from build123d import *

# Parameters (mm, degrees)
F0_R     = 10
F0_W     = 5
F0_H     = 8
F0_W_2   = 8
F0_H_2   = 5
F0_R_2   = 5
F1_DEPTH = 25


with BuildPart() as f1:
    # F0 (on Front) → F1 (new body)
    with BuildSketch(Plane.XZ):
        with BuildLine():
            ThreePointArc((60.975433, 96.400047), (60.980972, 96.732847), (60.982819, 97.065687))
            ThreePointArc((60.982819, 97.065687), (35.755982, 126.683535), (2.501691, 106.49041))
            ThreePointArc((2.501691, 106.49041), (2.393928, 106.15023), (2.285558, 105.810243))
            ThreePointArc((2.285558, 105.810243), (4.350114, 83.256305), (21.59361, 68.572833))
            ThreePointArc((21.59361, 68.572833), (48.295056, 72.564944), (60.975433, 96.400047))
        make_face()
        with Locations((30.982819, 97.065687)):
            Circle(F0_R, mode=Mode.SUBTRACT)
        with BuildLine():
            ThreePointArc((2.285558, 105.810243), (2.393928, 106.15023), (2.501691, 106.49041))
            ThreePointArc((2.501691, 106.49041), (2.391602, 106.150969), (2.285558, 105.810243))
        make_face()
        with BuildLine():
            ThreePointArc((-2.732649, -90.243404), (53.726427, -5.320256), (60.975433, 96.400047))
            ThreePointArc((60.975433, 96.400047), (48.295056, 72.564944), (21.59361, 68.572833))
            ThreePointArc((21.59361, 68.572833), (4.350114, 83.256305), (2.285558, 105.810243))
            ThreePointArc((2.285558, 105.810243), (-33.312028, 40.206629), (-90.483698, -7.776936))
            ThreePointArc((-90.483698, -7.776936), (-60.597191, -3.648374), (-33.776396, -17.46479))
            ThreePointArc((-33.776396, -17.46479), (-23.661975, -19.395325), (-14.685962, -14.349569))
            ThreePointArc((-14.685962, -14.349569), (-0.249152, -19.279648), (-7.475156, -32.715124))
            ThreePointArc((-7.475156, -32.715124), (-14.965806, -40.251179), (-25.569357, -40.934313))
            ThreePointArc((-25.569357, -40.934313), (-34.054638, -44.449031), (-37.569357, -52.934313))
            ThreePointArc((-37.569357, -52.934313), (-34.054638, -61.419594), (-25.569357, -64.934313))
            ThreePointArc((-25.569357, -64.934313), (-14.965806, -65.617446), (-7.475156, -73.153501))
            ThreePointArc((-7.475156, -73.153501), (0.078463, -80.260328), (-2.732649, -90.243404))
        make_face()
        with BuildLine():
            ThreePointArc((-3.124438, -90.590489), (-2.92843, -90.417074), (-2.732649, -90.243404))
            ThreePointArc((-2.732649, -90.243404), (0.078463, -80.260328), (-7.475156, -73.153501))
            ThreePointArc((-7.475156, -73.153501), (-14.965806, -65.617446), (-25.569357, -64.934313))
            ThreePointArc((-25.569357, -64.934313), (-34.054638, -61.419594), (-37.569357, -52.934313))
            ThreePointArc((-37.569357, -52.934313), (-34.054638, -44.449031), (-25.569357, -40.934313))
            ThreePointArc((-25.569357, -40.934313), (-14.965806, -40.251179), (-7.475156, -32.715124))
            ThreePointArc((-7.475156, -32.715124), (-0.249152, -19.279648), (-14.685962, -14.349569))
            ThreePointArc((-14.685962, -14.349569), (-23.661975, -19.395325), (-33.776396, -17.46479))
            ThreePointArc((-33.776396, -17.46479), (-60.597191, -3.648374), (-90.483698, -7.776936))
            ThreePointArc((-90.483698, -7.776936), (-92.822542, -9.066422), (-95.178396, -10.324562))
            ThreePointArc((-95.178396, -10.324562), (-108.31989, -83.842194), (-33.776396, -88.403835))
            ThreePointArc((-33.776396, -88.403835), (-23.661975, -86.4733), (-14.685962, -91.519056))
            ThreePointArc((-14.685962, -91.519056), (-8.756822, -92.902215), (-3.124438, -90.590489))
        make_face()
        Polygon((-80.882925, -83.436465), (-83.382925, -87.766593), (-90.311128, -83.766593), (-87.811128, -79.436465), align=None, mode=Mode.SUBTRACT)
        Polygon((-94.544293, -73.41708), (-98.87442, -75.91708), (-102.87442, -68.988877), (-98.544293, -66.488877), align=None, mode=Mode.SUBTRACT)
        with Locations((-103.865692, -53.909354)):
            Rectangle(F0_W, F0_H, mode=Mode.SUBTRACT)
        with Locations((-68.04214, -87.782824)):
            Rectangle(F0_W_2, F0_H_2, mode=Mode.SUBTRACT)
        Polygon((-48.534414, -78.461424), (-46.034414, -82.791551), (-52.962617, -86.791551), (-55.462617, -82.461424), align=None, mode=Mode.SUBTRACT)
        with BuildLine():
            ThreePointArc((-49.243461, -55.934313), (-89.017181, -52.934313), (-49.243461, -49.934313))
            Line((-49.243461, -49.934313), (-56.243461, -49.934313))
            Line((-56.243461, -49.934313), (-56.243461, -55.934313))
            Line((-56.243461, -55.934313), (-49.243461, -55.934313))
        make_face(mode=Mode.SUBTRACT)
        Polygon((-99.519334, -41.068569), (-103.849461, -38.568569), (-99.849461, -31.640366), (-95.519334, -34.140366), align=None, mode=Mode.SUBTRACT)
        Polygon((-89.499949, -27.407201), (-91.999949, -23.077074), (-85.071746, -19.077074), (-82.571746, -23.407201), align=None, mode=Mode.SUBTRACT)
        with Locations((-69.992223, -18.085801)):
            Rectangle(F0_W_2, F0_H_2, mode=Mode.SUBTRACT)
        Polygon((-57.151438, -22.43216), (-54.651438, -18.102033), (-47.723235, -22.102033), (-50.223235, -26.43216), align=None, mode=Mode.SUBTRACT)
        with Locations((-9.557397, -82.934313)):
            Circle(F0_R_2, mode=Mode.SUBTRACT)
        with Locations((-9.557397, -22.934313)):
            Circle(F0_R_2, mode=Mode.SUBTRACT)
        with BuildLine():
            ThreePointArc((-3.124438, -90.590489), (-2.926272, -90.41951), (-2.732649, -90.243404))
            ThreePointArc((-2.732649, -90.243404), (-2.92843, -90.417074), (-3.124438, -90.590489))
        make_face()
        with BuildLine():
            ThreePointArc((-95.178396, -10.324562), (-92.822542, -9.066422), (-90.483698, -7.776936))
            ThreePointArc((-90.483698, -7.776936), (-92.865091, -8.988014), (-95.178396, -10.324562))
        make_face()
    extrude(amount=F1_DEPTH)


solid = f1.part
Could you check a few things on this model? Use its own coordinates, in mm. A direction names the side the tool comes from. Give positions to 0.01 mm unless a question says otherwise; leave off trailing zeros. Order: outer loops, then holes, each group sorted by start corner. A loop starts at its lowest first (then second) coordinate and runs counter-clockwise, first axis right, second up. Notation, with made-up numbers: M -19.75,78 L -9.75,78 A21 cw -9.75,95 Z; hole C 21.25,69.25 d6. An arc over 180 degrees is marked long. One line per question, with ' | ' between items.
1. For faces 1 (the face through (-92.83, -12.32, -8.97)), 2 (the face through (-72.042, -12, -88)), which set-ups out of +Z, -Z, +X, -X, +Y, -Y let a thin tool reach every point of the face, with its end or its side?
Results:
face 1: +Z, -X, +Y, -Y | face 2: +Y, -Y
2. I'm going to push flat-ended pins straight in: pin 1 (12 mm diameter, centred on x = 30.98, z = 97.07, fed in from +Y); pin 2 (6 mm diameter, centred on x = -92.5, y = -10.5, fed in from +Z); pin 3 (2.5 mm diameter, centred on y = -6.5, z = -87.5, fed in from -X); pin 4 (9 mm diameter, centred on x = -66.5, y = -18.5, fed in from -Z). Where does each tip first touch, or does it pass through?
Results:
pin 1: through | pin 2: z = -7.22 | pin 3: x = -106.3 | pin 4: z = -102.93
3. We'd pull the mould along Z, two halves only. Please class faces 3 (the face through (-85.99, -12.32, -25.38)), 4 (the face through (-23.81, -12.32, -86.45)), 5 (the face through (36.34, -12.325, 126.583)): +Z half, -Z half, draft (parallel to the pull), parting line (faces both ways), or undercut.
Results:
face 3: undercut | face 4: -Z half | face 5: +Z half
4. I want a section at D-D (y = -7.25). Give the number of separate pieces and of enclosed holes in the cut face, and give its area (3 significant figures).
Results:
separate pieces: 1 | enclosed holes: 13 | area: 21,800 mm²
5. If I drill on line 1 (X direction, y = -2, z = -82); line 2 (Z direction, x = -7, y = -6); line 3 (X direction, y = -4.5, z = -83), over which ranges is the centre line in solid material (lowest first)?
Results:
line 1: -109.7 to -89.29, -83.37 to -54.66, -46.49 to -14.47, -4.65 to 6 | line 2: -92.6 to -87.23, -78.64 to -27.23, -18.64 to 82.09 | line 3: -108.97 to -89.87, -81.64 to -55.15, -46.4 to -14.56, -4.56 to 5
6. I want a section at C-C (z = 19). List the corners of the cut face in (x, y) for me, and give its area (3 significant figures).
Results:
outline: M -53.38,-25 L 60.35,-25 L 60.35,0 L -53.38,0 Z | area: 2,840 mm²
7. I want a section at A-A (x = 33). List the corners of the cut face in (y, z) for me.
Results:
outline: M -25,-48.37 L 0,-48.37 L 0,87.27 L -25,87.27 Z; M -25,106.86 L 0,106.86 L 0,127 L -25,127 Z
8. I want a section at B-B (x = -11). List the corners of the cut face in (y, z) for me, and give its area (3 significant figures).
Results:
outline: M -25,-92.83 L 0,-92.83 L 0,-87.72 L -25,-87.72 Z; M -25,-78.15 L 0,-78.15 L 0,-27.72 L -25,-27.72 Z; M -25,-18.15 L 0,-18.15 L 0,74.01 L -25,74.01 Z | area: 3,690 mm²
